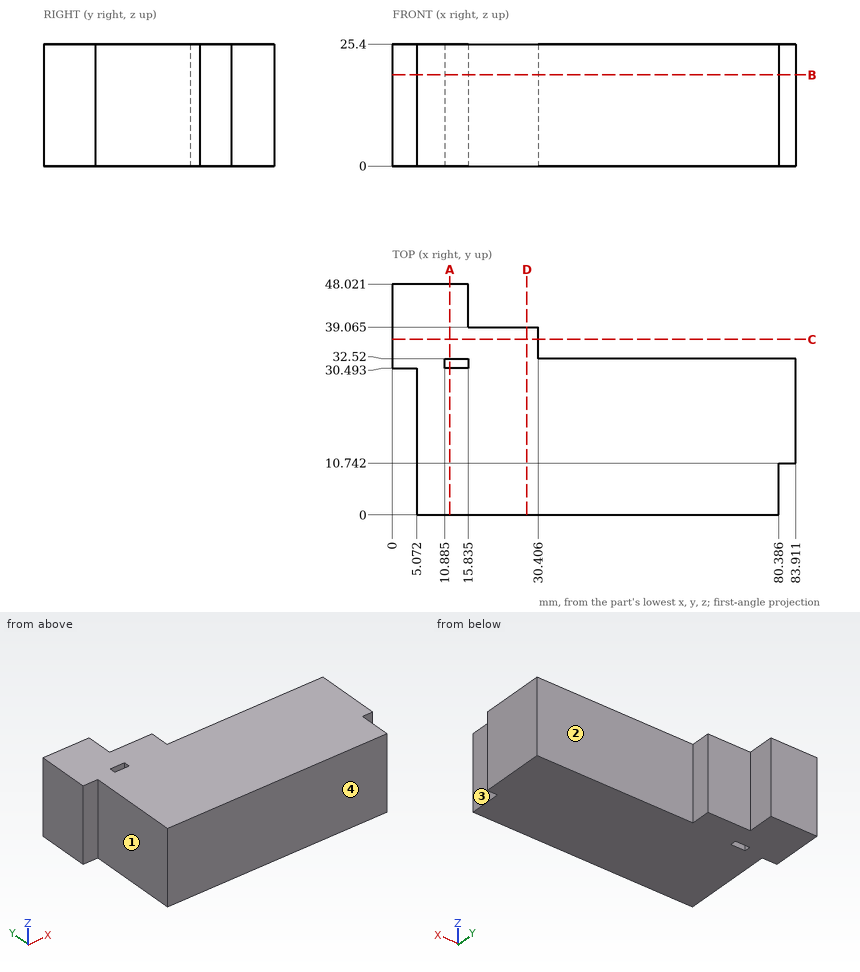
Could you check a few things on this drawing? It's one solid part, dimensions in mm from its lowest x, y, z. A direction names the side the tool comes from. Give positions to 0.01 mm unless a question says otherwise; leave off trailing zeros. Order: outer loops, then holes, each group sorted by start corner. A loop starts at its lowest first (then second) coordinate and runs counter-clockwise, first axis right, second up. Notation, with made-up numbers: (-8.5, 23.5) - (-0.5, 23.5) arc R7 ccw to (-0.5, 29.5) - close; hole circle Ø5 at (-38, -13.75). An arc over 180 degrees is marked (long way). One line per item, written item: value. Start each with the question number.
1. For the marked faces 1, 2, 3 and 4, which set-ups out of +Z, -Z, +X, -X, +Y, -Y let a thin tool reach every point of the face, with its end or its side?
2. Imagine slicing it at A-A on x = 12. List the corners of the cut face in (y, z) for me.
3. For P1, Ø2.5, axis at x = 2.5, z = 13.5, coming from the -Y side; P2, Ø1.5, axis at x = 34, y = 25, coming from the -Z side; P3, Ø8.5, axis at y = 6, z = 9.5, coming from the +X side; P4, Ø7.5, axis at x = 20, z = 16, coming from the +Y side (1 decimal), each with a flat end and sliding along its axis, tell me the tip position at first contact or that it passes through.
4. If I drill on probe 1 along X at (y, z) = (32, 23.5) (1 decimal); probe 2 along Y at (x, z) = (24.5, 7.75) (1 decimal); probe 3 along Y at (x, z) = (54, 18.25), over which ranges is the centre line in solid material (lowest first)?
5. Imagine slicing it at B-B on z = 19. List the corners of the cut face in (x, y) for me (1 decimal), plus the area to 3 significant figures.
6. Imagine slicing it at C-C on y = 36.5. List the corners of the cut face in (x, z) for me, plus the area to 3 significant figures.
7. Imagine slicing it at D-D on x = 28. List the corners of the cut face in (y, z) for me (1 decimal).
Values:
1. face 1: +Z, -Z, -X, -Y
1. face 2: +Z, -Z, +X, +Y
1. face 3: +Z, -Z, +X, -Y
1. face 4: +Z, -Z, +X, -X, -Y
2. outline: (0, 0) - (30.49, 0) - (30.49, 25.4) - (0, 25.4) - close; (32.52, 0) - (48.02, 0) - (48.02, 25.4) - (32.52, 25.4) - close
3. P1: y = 30.49
3. P2: z = 0
3. P3: x = 80.39
3. P4: y = 39.1
4. probe 1: 0 to 10.9, 15.8 to 83.9
4. probe 2: 0 to 39.1
4. probe 3: 0 to 32.52
5. outline: (0, 30.5) - (5.1, 30.5) - (5.1, 0) - (80.4, 0) - (80.4, 10.7) - (83.9, 10.7) - (83.9, 32.5) - (30.4, 32.5) - (30.4, 39.1) - (15.8, 39.1) - (15.8, 48) - (0, 48) - close; hole (10.9, 30.5) - (15.8, 30.5) - (15.8, 32.5) - (10.9, 32.5) - close
5. area: 2,870 mm²
6. outline: (0, 0) - (30.41, 0) - (30.41, 25.4) - (0, 25.4) - close
6. area: 772 mm²
7. outline: (0, 0) - (39.1, 0) - (39.1, 25.4) - (0, 25.4) - close
